The drawing under review shows one solid part. Ordinate dimensions are in mm from its lowest x, y, z. A direction names the side the tool comes from. Give positions to 0.01 mm unless a question says otherwise; leave off trailing zeros. Order: outer loops, then holes, each group sorted by start corner. A loop starts at its lowest first (then second) coordinate and runs counter-clockwise, first axis right, second up. Notation, with made-up numbers: (-19.75, 16.5) - (30.25, 16.5) arc R17 ccw to (30.25, 20.5) - close; hole circle Ø4 at (19.25, 28.25). An arc over 180 degrees is marked (long way). Use CSV: the item, a comma, the result in double quotes.
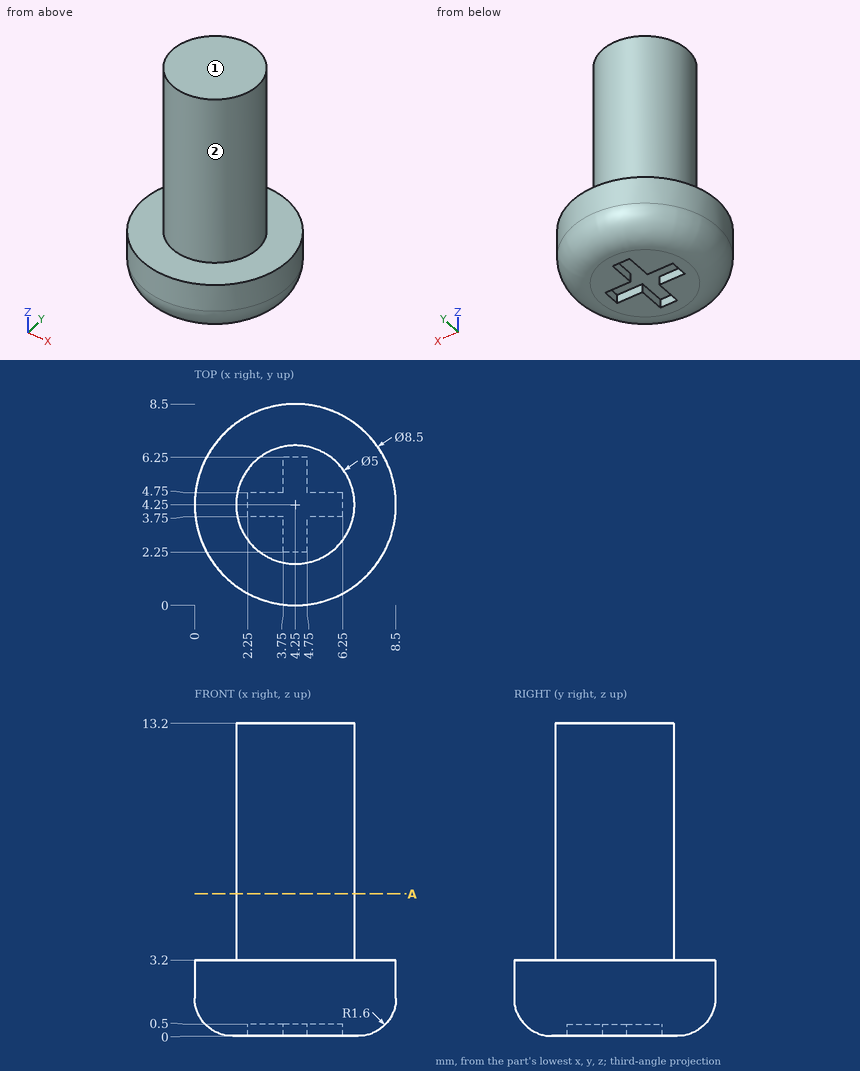
Item 1: Take a section at A-A, the plane z = 6. Give the boundary of the cut face in (x, y), and give its area (3 significant figures).
Results list:
outline,"circle Ø5 at (4.25, 4.25)"
area,"19.6 mm2"
Item 2: Clearance check with flat-ended pins moving along their axes: pin 1 (0.6 mm diameter, centred on x = 4.5, z = 0.5, fed in from -Y); pin 2 (2 mm diameter, centred on x = 7.5, z = 10.5, fed in from -Y); pin 3 (0.6 mm diameter, centred on y = 4.5, z = 0.5, fed in from -X). State where each tip first meets the part, or that it passes through.
Results list:
pin 1,"stops at y = 0.22"
pin 2,"stops at y = 3.16"
pin 3,"stops at x = 0.22"
Item 3: Wall thickness on L1, parallel to Z at x = 2.25, y = 2.5; L2, parallel to Z at x = 5.75, y = 4.25; L3, parallel to X at y = 5.75, z = 9.75: over which ranges is each line inside the solid? List them lowest first.
Results list:
L1,"z = 0 to 3.2"
L2,"z = 0.5 to 13.2"
L3,"x = 2.25 to 6.25"
Item 4: Tool access review of the marked faces 1 and 2: name each direction out of +Z, -Z, +X, -X, +Y, -Y from which nothing blocks a thin tool from reaching the whole face with its end or side.
Results list:
face 1,"+Z, +X, -X, +Y, -Y"
face 2,"+Z"
